Source: CAD feature listing. Evaluate the final solid. Frame: model axes, mm. Face numbers are marked on the shaded views. A direction names the side the tool comes from. Give positions to 0.01 mm unless a question says otherwise; leave off trailing zeros. Write each loop counter-clockwise with the first axis right and the second up, starting at its lowest first coordinate (ties: lowest second). Pieces come first, ordered by that corner, then holes. Notation, with made-up numbers: M 47,-21 L 75,-21 A34 cw 75,9 Z; hole C 42.5,55 d9. An arc over 180 degrees is marked long. Answer as a JSON object with one key per item and string values. Group by question number.
```python
from build123d import *

# Parameters (mm, degrees)
ESQUISSE1_R        = 1.25
ESQUISSE1_R_2      = 1.5
BOSS_EXTRU_1_DEPTH = 25


with BuildPart() as part:
    # Esquisse1 → Boss.-Extru.1 (new, symmetric)
    with BuildSketch(Plane.XY):
        with BuildLine():
            Line((-2.571150439, 3.064177772), (6.350420085, 10.550264309))
            ThreePointArc((6.350420085, 10.550264309), (16.35179369, 14.692968898), (26.92059706, 12.349921601))
            Line((26.92059706, 12.349921601), (42.311288741, 3.464101615))
            ThreePointArc((42.311288741, 3.464101615), (43.775390357, -2), (38.311288741, -3.464101615))
            Line((38.311288741, -3.464101615), (22.92059706, 5.42171837))
            ThreePointArc((22.92059706, 5.42171837), (17.049039632, 6.723411313), (11.492720963, 4.421908764))
            Line((11.492720963, 4.421908764), (2.571150439, -3.064177772))
            ThreePointArc((2.571150439, -3.064177772), (-3.064177772, -2.571150439), (-2.571150439, 3.064177772))
        make_face()
        Circle(ESQUISSE1_R, mode=Mode.SUBTRACT)
        with Locations((40.311288741, 0)):
            Circle(ESQUISSE1_R_2, mode=Mode.SUBTRACT)
    extrude(amount=BOSS_EXTRU_1_DEPTH, both=True)

    # Esquisse4 → Enlèvement de matière-Révolution1 (revolve, cut)
    with BuildSketch(Plane(origin=(0, 0, 0), x_dir=(1, 0, 0), z_dir=(0, 1, 0))):
        with BuildLine():
            Line((80, 17.5), (80, 25))
            Line((80, 25), (5.633213888, 25))
            ThreePointArc((5.633213888, 25), (6.414996134, 24.93850347), (7.177547622, 24.755526608))
            Line((7.177547622, 24.755526608), (28.766955008, 17.744473392))
            ThreePointArc((28.766955008, 17.744473392), (29.529506495, 17.56149653), (30.311288741, 17.5))
            Line((30.311288741, 17.5), (80, 17.5))
        make_face()
        with BuildLine():
            Line((0, 21), (5, 21))
            ThreePointArc((5, 21), (7.5, 20.330127019), (9.330127019, 18.5))
            Line((9.330127019, 18.5), (18.567731326, 2.5))
            ThreePointArc((18.567731326, 2.5), (19.237604307, 0), (18.567731326, -2.5))
            Line((18.567731326, -2.5), (9.330127019, -18.5))
            ThreePointArc((9.330127019, -18.5), (7.5, -20.330127019), (5, -21))
            Line((5, -21), (0, -21))
            Line((0, -21), (0, 21))
        make_face()
        with BuildLine():
            Line((30.311288741, -17.5), (80, -17.5))
            Line((80, -17.5), (80, -25))
            Line((80, -25), (5.633213888, -25))
            ThreePointArc((5.633213888, -25), (6.414996134, -24.93850347), (7.177547622, -24.755526608))
            Line((7.177547622, -24.755526608), (28.766955008, -17.744473392))
            ThreePointArc((28.766955008, -17.744473392), (29.529506495, -17.56149653), (30.311288741, -17.5))
        make_face()
    revolve(axis=Axis((0, 0, 25), (0, 0, -1)), mode=Mode.SUBTRACT)


solid = part.part
```
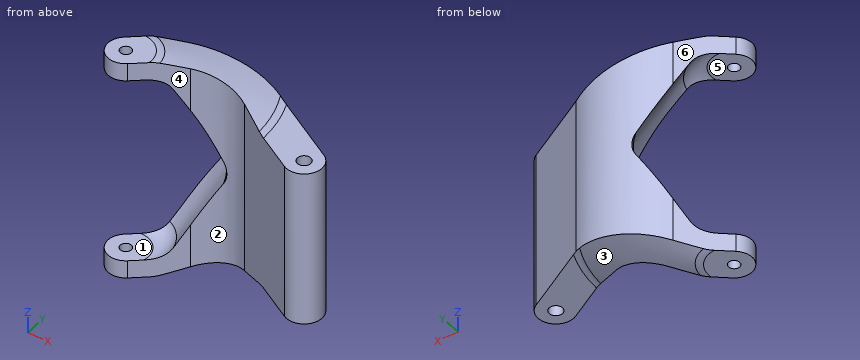
(1) Section A-A, the plane z = 15. Return loops of the section in (x, y).
(2) Section B-B, the plane z = -8. Return loops of the section in (x, y), plus the area to 3 significant figures.
(3) Access query for the marked faces 4, 5 and 6. Directions: +Z, -Z, +X, -X, +Y, -Y. A direction counts if a zero-diameter tool reaches every point of the face in a straight line with its end or side. Return the directions, or none.
(4) Contact query for flat-ended pins moving along their axis: pin 1 Ø10 at (x, z) = (6, 15.5) entering from -Y; pin 2 Ø4.5 at (x, y) = (39, 7.5) entering from +Z; pin 3 Ø10 at (y, z) = (11, 17) entering from +X; pin 4 Ø2 at (x, y) = (0, 0) entering from -Z. Output: stop coordinate, or through.
(5) Ray query, L1, parallel to Z at x = 33, y = 8.25; L2, parallel to Z at x = 3, y = 4.5; L3, parallel to X at y = 0, z = 23.5. Return the intervals inside material, ascending. Write a range as [from, to].
(6) Pull-direction query (X, two-part tool) for the marked faces 1, 2 and 3; classes: pulls with the +X half, pulls with the -X half, needs draft (parallel to the pull), parting line crosses it, or undercut.
Reported:
{
 "1": {"outline": "M 5.57,9.89 A11.35 cw 10.71,3.76 L 11.49,4.42 A10 cw 22.92,5.42 L 38.31,-3.46 A4 ccw 42.31,3.46 L 26.92,12.35 A18 ccw 6.35,10.55 Z; hole C 40.31,0 d3"},
 "2": {"outline": "M 9.07,12.44 A15.39 cw 14.16,6.03 A10 cw 22.92,5.42 L 38.31,-3.46 A4 ccw 42.31,3.46 L 26.92,12.35 A18 ccw Z; hole C 40.31,0 d3", "area": "268 mm2"},
 "3": {"face 4": "+Z, -Z, -Y", "face 5": "-X, -Y", "face 6": "+Z, -Z, -X, +Y"},
 "4": {"pin 1": "stops at y = 1.11", "pin 2": "stops at z = 17.5", "pin 3": "stops at x = 37.92", "pin 4": "passes through"},
 "5": {"L1": "z = [-17.5, 17.5]", "L2": "z = [-25, -20.98], [20.98, 25]", "L3": "x = [-4, -1.25], [1.25, 6.22]"},
 "6": {"face 1": "needs draft", "face 2": "undercut", "face 3": "pulls with the +X half"}
}
